Geometry check sheet. Reference: the model listing, model coordinates, mm. Face numbers are marked on the shaded views. A direction names the side the tool comes from. Coordinates: 2 decimals unless noted, no trailing zeros. Write each loop counter-clockwise with the first axis right and the second up, starting at its lowest first coordinate (ties: lowest second). Pieces come first, ordered by that corner, then holes. Notation, with made-up numbers: (-39.75, 89) -> (-4.75, 89) arc R23 cw to (-4.75, 101) -> close; hole circle Ø11 at (16, 78.5). An arc over 180 degrees is marked (long way). Use a Markdown table: item, result.
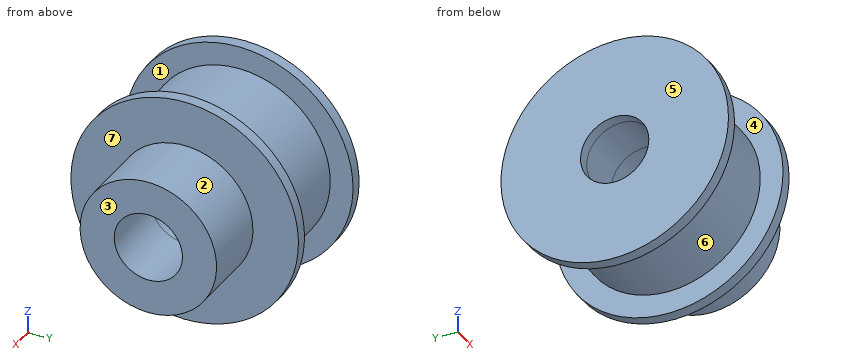
Autodesk Inventor part; units mm, degrees
ref_plane "YZ Plane" through (0, 0, 0) normal (1, 0, 0) x (0, 1, 0)
ref_plane "XZ Plane" through (0, 0, 0) normal (0, 1, 0) x (-1, 0, 0)
ref_plane "XY Plane" through (0, 0, 0) normal (0, 0, 1) x (1, 0, 0)
sketch "Sketch1" plane through (0, 0, 0) normal (1, 0, 0) x (0, 1, 0)
  circle A0 centre (0, 0) radius 12.7
  circle A1 centre (0, 0) radius 4.7625
  dimension "d0" = 25.4
  dimension "d2" = 9.525
extrude "Extrusion1" add sketch "Sketch1" along normal mid plane 12.7
sketch "Sketch2" plane through (6.35, 0, 0) normal (1, 0, 0) x (0, 0, -1)
  circle A0 centre (0, 0) radius 15.875
  circle A1 centre (0, 0) radius 12.7 construction
  circle A2 centre (0, 0) radius 4.7625
  dimension "d6" = 3.175
extrude "Extrusion2" add sketch "Sketch2" along normal blind 1.5875
sketch "Sketch3" plane through (-6.35, 0, 0) normal (-1, 0, 0) x (0, 0, 1)
  circle A0 centre (0, 0) radius 15.875
  circle A1 centre (0, 0) radius 4.7625
extrude "Extrusion3" add sketch "Sketch3" along normal blind 1.5875
sketch "Sketch4" plane through (7.9375, 0, 0) normal (1, 0, 0) x (0, 0, -1)
  circle A0 centre (0, 0) radius 4.7625
  circle A1 centre (0, 0) radius 9.525
  dimension "d11" = 4.7625
extrude "Extrusion4" add sketch "Sketch4" along normal blind 9.525
properties part number "pulley XL 1in" material "Aluminum 6061"
Item 1: Mould release check, pull along X, two halves, no side actions. Record for the marked faces 4, 5, 6 and 7: +X half, -X half, draft (parallel to the pull), parting line (faces both ways), or undercut.
Answer block:
| item | result |
|---|---|
| face 4 | undercut |
| face 5 | -X half |
| face 6 | undercut |
| face 7 | +X half |
Item 2: Section check D-D on z = -8. Record the boundary of the cut face in (x, y).
Answer block:
| item | result |
|---|---|
| outline | (-7.94, -13.71) -> (-6.35, -13.71) -> (-6.35, -9.86) -> (6.35, -9.86) -> (6.35, -13.71) -> (7.94, -13.71) -> (7.94, -5.17) -> (17.46, -5.17) -> (17.46, 5.17) -> (7.94, 5.17) -> (7.94, 13.71) -> (6.35, 13.71) -> (6.35, 9.86) -> (-6.35, 9.86) -> (-6.35, 13.71) -> (-7.94, 13.71) -> close |
Item 3: Section check C-C on x = -4. Record the boundary of the cut face in (y, z) (1 decimal).
Answer block:
| item | result |
|---|---|
| outline | circle Ø25.4 at (0, 0); hole circle Ø9.5 at (0, 0) |
Item 4: Depth check by flat-ended pin: P1, Ø8, axis at x = 12.5, y = -8, coming from the +Z side; P2, Ø3, axis at y = -9.5, z = -7, coming from the +X side; P3, Ø4, axis at x = 2.5, y = -9.5, coming from the +Z side. Enter the tip coordinate at first touch or a pass-through.
Answer block:
| item | result |
|---|---|
| P1 | stops at z = 8.64 |
| P2 | stops at x = 7.94 |
| P3 | stops at z = 10.25 |
Item 5: Tool access check on the marked faces 1, 2 and 3. Record the directions out of +Z, -Z, +X, -X, +Y, -Y that give a thin tool (end or side, any length) a straight path to the whole face; none if there is none.
Answer block:
| item | result |
|---|---|
| face 1 | none |
| face 2 | +X |
| face 3 | +Z, -Z, +X, +Y, -Y |
Item 6: Thickness scan on L1, parallel to Y at x = 6.7, z = 0 (1 decimal); L2, parallel to X at y = 12, z = -8; L3, parallel to Y at x = -2, z = -4. Record the ranges inside material, lowest first. Write a range as [from, to].
Answer block:
| item | result |
|---|---|
| L1 | y = [-15.9, -4.8], [4.8, 15.9] |
| L2 | x = [-7.94, -6.35], [6.35, 7.94] |
| L3 | y = [-12.05, -2.58], [2.58, 12.05] |
